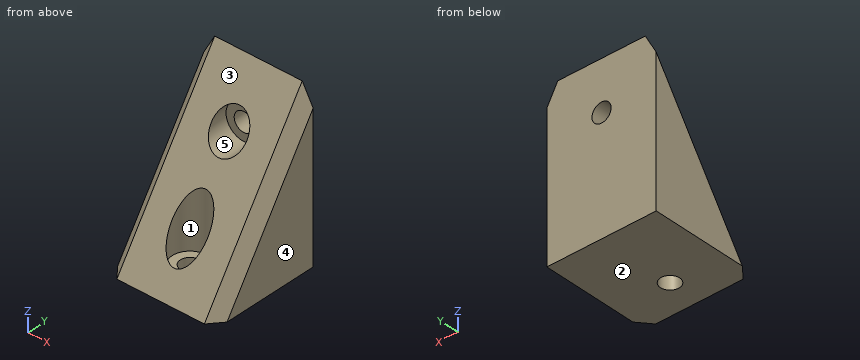
```python
from build123d import *

# Parameters (mm, degrees)
F0_W     = 20
F0_H     = 30
F1_DEPTH = 20
F2_R     = 3.25
F2_R_2   = 1.75
F3_DEPTH = 17
F4_DEPTH = 20.001
F7_DEPTH = 20.001
F5_R     = 3.25
F5_R_2   = 1.75
F8_DEPTH = 27
F9_DEPTH = 30.001
F10_SIZE = 2


with BuildPart() as f1:
    # F0 (on Front) → F1 (new body)
    with BuildSketch(Plane.XZ):
        with Locations((10, 15)):
            Rectangle(F0_W, F0_H)
    extrude(amount=F1_DEPTH)

    # F2 (on face) → F3 (cut)
    with BuildSketch(Plane.XZ.offset(20)):
        with Locations((10, 21)):
            Circle(F2_R)
        with Locations((10, 21)):
            Circle(F2_R_2, mode=Mode.SUBTRACT)
    extrude(amount=-F3_DEPTH, mode=Mode.SUBTRACT)

    # F4 (cut, through all): a face of the model
    f4_faces = [f1.faces().sort_by_distance(p)[0] for p in [
        (10, -20, 21),
    ]]
    extrude(f4_faces, amount=-F4_DEPTH, mode=Mode.SUBTRACT)

    # F6 (on face) → F7 (cut, through all)
    with BuildSketch(Plane(origin=(0, 0, 0), x_dir=(0, -1, 0), z_dir=(-1, 0, 0))):
        Polygon((20, 30), (0, 30), (20, 0), align=None)
    extrude(amount=-F7_DEPTH, mode=Mode.SUBTRACT)

    # F5 (on face) → F8 (cut)
    with BuildSketch(Plane.XY.offset(30)):
        with Locations((10, -14)):
            Circle(F5_R)
        with Locations((10, -14)):
            Circle(F5_R_2, mode=Mode.SUBTRACT)
    extrude(amount=-F8_DEPTH, mode=Mode.SUBTRACT)

    # F5 (on face) → F9 (cut, through all)
    with BuildSketch(Plane.XY.offset(30)):
        with Locations((10, -14)):
            Circle(F5_R_2)
    extrude(amount=-F9_DEPTH, mode=Mode.SUBTRACT)

    # F10
    f10_edges = [f1.edges().sort_by_distance(p)[0] for p in [
        (0, -10, 15),
        (20, -10, 15),
    ]]
    chamfer(f10_edges, length=F10_SIZE)


solid = f1.part
```
The model under review builds one solid part; all positions refer to its coordinate system, in mm. Face numbers are marked on the shaded views. A direction names the side the tool comes from. Round coordinates to 2 decimals unless told otherwise and drop trailing zeros. Order: outer loops, then holes, each group sorted by start corner. A loop starts at its lowest first (then second) coordinate and runs counter-clockwise, first axis right, second up. Notation, with made-up numbers: (7.25, 57) - (62.25, 57) arc R24 cw to (62.25, 73) - close; hole circle Ø9 at (84.25, 7). An arc over 180 degrees is marked (long way). Answer in a Markdown table with one row per item.
(1) Mouldability with a two-part tool opening along X and no side actions: class the marked faces 3, 4 and 5 as released by +X, released by -X, zero draft, split by the parting line, or undercut.
Result set:
| item | result |
|---|---|
| face 3 | zero draft |
| face 4 | released by +X |
| face 5 | undercut |
(2) Machinability: for the marked faces 1 and 2, which of the approach directions +Z, -Z, +X, -X, +Y, -Y give a long, thin tool a straight path to every point of the face, cutting with its end or side? Answer none if there is none.
Result set:
| item | result |
|---|---|
| face 1 | +Z |
| face 2 | -Z, +X, -X, +Y, -Y |
(3) Take a section at D-D on x = 6. Write out the cut boundary in (y, z), plus the area to 3 significant figures.
Result set:
| item | result |
|---|---|
| outline | (-20, 0) - (0, 0) - (0, 30) - close |
| area | 300 mm2 |
(4) Clearance check with flat-ended pins moving along their axes: P1, Ø4, axis at x = 10, z = 21, coming from the -Y side; P2, Ø10, axis at x = 17, z = 21.5, coming from the -Y side; P3, Ø1.5, axis at x = 16.5, z = 19.5, coming from the -Y side; P4, Ø4, axis at y = -15, z = 14.5, coming from the +X side (3 decimals). State where each tip first meets the part, or that it passes through.
Result set:
| item | result |
|---|---|
| P1 | stops at y = -3 |
| P2 | stops at y = -9 |
| P3 | stops at y = -7.5 |
| P4 | passes through |
(5) Take a section at C-C on z = 7. Write out the cut boundary in (x, y), plus the area to 3 significant figures.
Result set:
| item | result |
|---|---|
| outline | (0, -12.93) - (2, -15.33) - (7.04, -15.33) arc R3.25 cw (long way) to (12.96, -15.33) - (18, -15.33) - (20, -12.93) - (20, 0) - (0, 0) - close |
| area | 277 mm2 |
(6) For line 1 (Z direction, x = 10, y = -2.4); line 2 (X direction, y = -14, z = 8.75); line 3 (Y direction, x = 10, z = 1.05), list the stretches that pass through material, from the lowest coordinate up. Write a range as from..to.
Result set:
| item | result |
|---|---|
| line 1 | z = 0..19.25, 22.75..26.4 |
| line 2 | x = 1.86..6.75, 13.25..18.14 |
| line 3 | y = -19.3..-15.75, -12.25..0 |
(7) Take a section at A-A on x = 10. Write out the cut boundary in (y, z) (3 decimals), plus the area to 4 significant figures.
Result set:
| item | result |
|---|---|
| outline | (-20, 0) - (-15.75, 0) - (-15.75, 3) - (-17.25, 3) - (-17.25, 4.125) - close; (-12.25, 0) - (0, 0) - (0, 19.25) - (-3, 19.25) - (-3, 17.75) - (-8.167, 17.75) - (-10.75, 13.875) - (-10.75, 3) - (-12.25, 3) - close; (-3.833, 24.25) - (-3, 24.25) - (-3, 22.75) - (0, 22.75) - (0, 30) - close |
| area | 220.5 mm2 |
(8) Take a section at B-B on y = -14. Write out the cut boundary in (x, z).
Result set:
| item | result |
|---|---|
| outline | (0, 0) - (8.25, 0) - (8.25, 3) - (6.75, 3) - (6.75, 9) - (2, 9) - (0, 5.39) - close; (11.75, 0) - (20, 0) - (20, 5.39) - (18, 9) - (13.25, 9) - (13.25, 3) - (11.75, 3) - close |
